```python
from build123d import *

# Parameters (mm, degrees)
SKETCH1_W               = 3
SKETCH1_H               = 12.5
SKETCH1_W_2             = 1
SKETCH1_H_2             = 1
CUT_EXTRUDE1_DEPTH      = 18.550618775
CUT_EXTRUDE1_DEPTH_BACK = 18.550618775
SKETCH1_4_W             = 1
SKETCH1_4_H             = 1


with BuildPart() as part:
    # Sketch1 → Revolve1 (revolve)
    with BuildSketch(Plane.XY, mode=Mode.PRIVATE) as revolve1_sk:
        Polygon((0, 12.5), (3, 12.5), (6.5, 14.950726384), (1, 14.950726384), (1, 13.950726384), (0, 13.950726384), align=None)
        with Locations((1.5, 6.25)):
            Rectangle(SKETCH1_W, SKETCH1_H)
        Polygon((0, -1.732050808), (0, 0), (3, 0), align=None)
        with Locations((0.5, 14.450726384)):
            Rectangle(SKETCH1_W_2, SKETCH1_H_2)
    revolve(revolve1_sk.sketch.rotate(Axis((0, 14.950726384, 0), (0, -1, 0)), 90), axis=Axis((0, 14.950726384, 0), (0, -1, 0)))

    # Sketch1_4 → Cut-Extrude1 (cut, two sides: drawn at the far end of the back side and taken through both)
    with BuildSketch(Plane.XY.offset(-CUT_EXTRUDE1_DEPTH_BACK)):
        with Locations((-0.5, 14.450726384)):
            Rectangle(SKETCH1_4_W, SKETCH1_4_H)
        with Locations((0.5, 14.450726384)):
            Rectangle(SKETCH1_4_W, SKETCH1_4_H)
    extrude(amount=CUT_EXTRUDE1_DEPTH + CUT_EXTRUDE1_DEPTH_BACK, mode=Mode.SUBTRACT)


solid = part.part
```
Geometry check sheet. Reference: the model listing, model coordinates, mm. A direction names the side the tool comes from. Give positions to 0.01 mm unless a question says otherwise; leave off trailing zeros. Write each loop counter-clockwise with the first axis right and the second up, starting at its lowest first coordinate (ties: lowest second). Pieces come first, ordered by that corner, then holes.
1) Section check B-B, the plane y = 13. Record the boundary of the cut face in (x, z), and give its area (3 significant figures).
2) Material ranges on L1, parallel to X at y = 14.25, z = -1; L2, parallel to Z at x = -1, y = 13.25; L3, parallel to Z at x = -0.75, y = 13.25, recorded low to high.
3) Access from +Z, -Z, +X, -X, +Y, -Y to the whole of each face (thin tool, end or side, straight path). Record for faces 4 (the flat face through (-1, 14.4, -0.1)), 5 (the flat face through (3, 14.951, 0)), 6 (the cylindrical face through (-0.9, 6.34, 2.86)).
4) Release check for a two-part mould opening along X. For faces 1 (the flat face through (-3, 14.951, 0)), 2 (the conical face through (-0.967, 12.653, 3.07)), 3 (the flat face through (0, 13.951, 0)) record: pulls with the +X half, pulls with the -X half, needs draft (parallel to the pull), parting line crosses it, or undercut.
5) Section check A-A, the plane y = 5.5. Record the boundary of the cut face in (x, z), and give its area (3 significant figures).
6) Gauge pin test, flat ends, axial feed: pin 1 (4 mm diameter, centred on y = 8, z = 3, fed in from +X); pin 2 (1.1 mm diameter, centred on y = 14.5, z = 2.5, fed in from +X); pin 3 (0.5 mm diameter, centred on y = 14.5, z = 0, fed in from -X). Record the tip position at first contact, or that the pin passes through.
Computed:
1. outline: circle Ø7.43 at (0, 0)
1. area: 43.3 mm2
2. L1: x = -5.41 to -1, 1 to 5.41
2. L2: z = -3.95 to 3.95
2. L3: z = -4 to 4
3. face 4: +Z, -Z, +Y
3. face 5: +Z, -Z, +X, -X, +Y
3. face 6: -Y
4. face 1: needs draft
4. face 2: parting line crosses it
4. face 3: undercut
5. outline: circle Ø6 at (0, 0)
5. area: 28.3 mm2
6. pin 1: stops at x = 2.83
6. pin 2: stops at x = 6.12
6. pin 3: stops at x = -6.21
